Geometry: final body of the model. Coordinates: model frame, mm. Face numbers are marked on the shaded views. A direction names the side the tool comes from. Coordinates: 2 decimals unless noted, no trailing zeros. Order: outer loops, then holes, each group sorted by start corner. A loop starts at its lowest first (then second) coordinate and runs counter-clockwise, first axis right, second up. Notation, with made-up numbers: M 18.5,-31.5 L 41.5,-31.5 A19 cw 41.5,-25.5 Z; hole C 42.25,1 d10. An arc over 180 degrees is marked long. One line per question, with ' | ' between items.
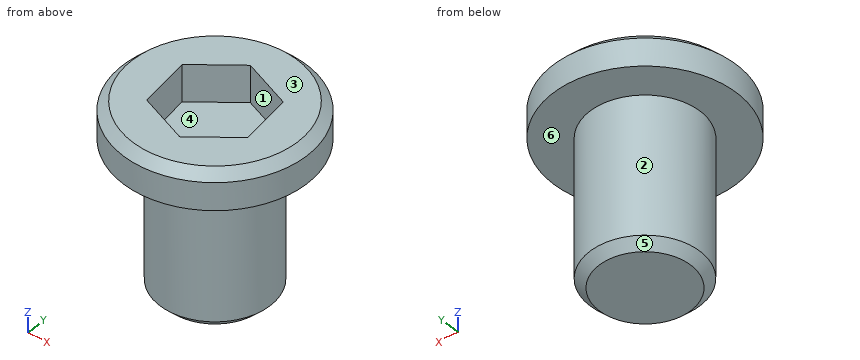
from build123d import *

# Parameters (mm, degrees)
F0_R     = 2.5
F1_DEPTH = 1
F2_R     = 1.5
F3_DEPTH = 4
F4_SIZE  = 0.25
F5_SIZE  = 0.25


with BuildPart() as f1:
    # F0 (on Top) → F1 (new body)
    with BuildSketch(Plane.XY):
        Circle(F0_R)
        Polygon((1.133814, 0.893196), (1.340438, -0.535313), (0.206624, -1.42851), (-1.133814, -0.893196), (-1.340438, 0.535313), (-0.206624, 1.42851), align=None, mode=Mode.SUBTRACT)
    extrude(amount=F1_DEPTH)

    # F2 (on face) → F3 (join)
    with BuildSketch(Plane(origin=(0, 0, 0), x_dir=(1, 0, 0), z_dir=(0, 0, -1))):
        Circle(F2_R)
    extrude(amount=F3_DEPTH)

    # F4
    f4_edges = [f1.edges().sort_by_distance(p)[0] for p in [
        (-2.5, 0, 1),
    ]]
    chamfer(f4_edges, length=F4_SIZE)

    # F5
    f5_edges = [f1.edges().sort_by_distance(p)[0] for p in [
        (-1.5, 0, -4),
    ]]
    chamfer(f5_edges, length=F5_SIZE)


solid = f1.part
1. Draft query along Y for the marked faces 4, 5 and 6. Return one class per face: pulls with the +Y half, pulls with the -Y half, needs draft (parallel to the pull), parting line crosses it, or undercut.
Response values:
face 4: undercut | face 5: parting line crosses it | face 6: needs draft
2. Material intervals for line 1 (Z direction, x = 0.75, y = -1.8); line 2 (Y direction, x = -0.85, z = 0.4); line 3 (Z direction, x = 0.5, y = -1), sorted ascending. Write a range as [from, to].
Response values:
line 1: z = [0, 1] | line 2: y = [-2.35, -1.01], [0.92, 2.35] | line 3: z = [-4, 0]
3. Pin query (flat end, axial travel): P1, Ø1, axis at x = 0.5, y = -0.5, coming from the +Z side; P2, Ø1, axis at x = 1.5, y = 1.5, coming from the -Z side. Return the tip coordinate at first contact, or that it passes through.
Response values:
P1: stops at z = 0 | P2: stops at z = 0
4. Section B-B, the plane y = 0. Output: boundary loops of the cut face in (x, z), and give its area (3 significant figures).
Response values:
outline: M -2.5,0 L -1.5,0 L -1.5,-3.75 L -1.25,-4 L 1.25,-4 L 1.5,-3.75 L 1.5,0 L 2.5,0 L 2.5,0.75 L 2.25,1 L 1.26,1 L 1.26,0 L -1.26,0 L -1.26,1 L -2.25,1 L -2.5,0.75 Z | area: 14.3 mm^2
5. Section C-C, the plane z = -1.5. Output: boundary loops of the cut face in (x, y).
Response values:
outline: C 0,0 d3
6. Section A-A, the plane x = 0. Output: boundary loops of the cut face in (y, z).
Response values:
outline: M -2.5,0 L -1.5,0 L -1.5,-3.75 L -1.25,-4 L 1.25,-4 L 1.5,-3.75 L 1.5,0 L 2.5,0 L 2.5,0.75 L 2.25,1 L 1.35,1 L 1.35,0 L -1.35,0 L -1.35,1 L -2.25,1 L -2.5,0.75 Z
7. Access query for the marked faces 1, 2 and 3. Directions: +Z, -Z, +X, -X, +Y, -Y. A direction counts if a zero-diameter tool reaches every point of the face in a straight line with its end or side. Return the directions, or none.
Response values:
face 1: +Z | face 2: -Z | face 3: +Z, +X, -X, +Y, -Y
